```python
from build123d import *

# Parameters (mm, degrees)
SKETCH1_W           = 22
SKETCH1_H           = 14
BOSS_EXTRUDE1_DEPTH = 40
BOSS_EXTRUDE2_DEPTH = 5
SKETCH3_R           = 3.25
CUT_EXTRUDE1_DEPTH  = 41
SKETCH4_W           = 1.2
SKETCH4_H           = 40
CUT_EXTRUDE2_DEPTH  = 0.8


with BuildPart() as part:
    # Sketch1 → Boss-Extrude1 (new body)
    with BuildSketch(Plane(origin=(0, 0, 0), x_dir=(1, 0, 0), z_dir=(0, 1, 0))):
        with Locations((11, 7)):
            Rectangle(SKETCH1_W, SKETCH1_H)
    extrude(amount=BOSS_EXTRUDE1_DEPTH)

    # Sketch2 → Boss-Extrude2 (add)
    with BuildSketch(Plane(origin=(0, 40, 0), x_dir=(1, 0, 0), z_dir=(0, 1, 0))):
        Polygon((22, 0), (22, 2), (2, 2), (2, 12), (22, 12), (22, 14), (0, 14), (0, 0), align=None)
    extrude(amount=BOSS_EXTRUDE2_DEPTH)

    # Sketch3 → Cut-Extrude1 (cut, through all)
    with BuildSketch(Plane(origin=(0, 40, 0), x_dir=(1, 0, 0), z_dir=(0, 1, 0))):
        with Locations((16.582903769, 7)):
            Circle(SKETCH3_R)
        Polygon((11.582903769, 7), (9.562177826, 10.5), (5.520725942, 10.5), (3.5, 7), (5.520725942, 3.5), (9.562177826, 3.5), align=None)
    extrude(amount=-CUT_EXTRUDE1_DEPTH, mode=Mode.SUBTRACT)

    # Sketch4 → Cut-Extrude2 (cut)
    with BuildSketch(Plane(origin=(22, 0, 0), x_dir=(0, 0, -1), z_dir=(1, 0, 0))):
        with Locations((7, 20)):
            Rectangle(SKETCH4_W, SKETCH4_H)
    extrude(amount=-CUT_EXTRUDE2_DEPTH, mode=Mode.SUBTRACT)


solid = part.part
```
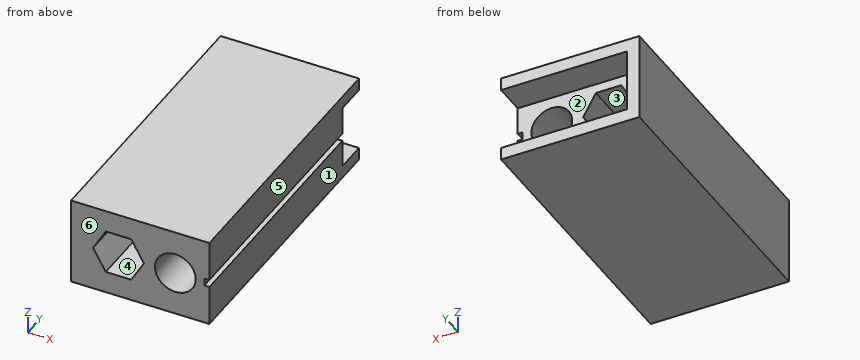
Could you check a few things on this model? Use its own coordinates, in mm. Face numbers are marked on the shaded views. A direction names the side the tool comes from. Give positions to 0.01 mm unless a question says otherwise; leave off trailing zeros. Loops run counter-clockwise (first coordinate to the right, second up) from the corner with the lowest first, then second, coordinate; pieces in that order, holes last. Notation, with made-up numbers: (61.25, -18.5) -> (85.25, -18.5) arc R15 ccw to (85.25, -4.5) -> close; hole circle Ø8 at (66, -6). An arc over 180 degrees is marked (long way). Put each result on its own line as item: value.
(1) I'm going to push flat-ended pins straight in: pin 1 Ø4 at (x, z) = (14.5, -5) entering from -Y; pin 2 Ø1.5 at (y, z) = (43.5, -4.5) entering from +X; pin 3 Ø0.6 at (y, z) = (24, -7) entering from +X; pin 4 Ø3 at (x, z) = (14.5, -5.5) entering from +Y. Where does each tip first touch, or does it pass through?
Computed:
pin 1: y = 0
pin 2: x = 2
pin 3: x = 21.2
pin 4: y = 40
(2) Imagine slicing it at B-B on x = 12.25. Write out the boundary of the cut face in (y, z).
Computed:
outline: (0, -14) -> (45, -14) -> (45, -12) -> (40, -12) -> (40, -2) -> (45, -2) -> (45, 0) -> (0, 0) -> close
(3) Imagine slicing it at A-A on y = 14.5. Write out the boundary of the cut face in (x, z).
Computed:
outline: (0, -14) -> (22, -14) -> (22, -7.6) -> (21.2, -7.6) -> (21.2, -6.4) -> (22, -6.4) -> (22, 0) -> (0, 0) -> close; hole (3.5, -7) -> (5.52, -10.5) -> (9.56, -10.5) -> (11.58, -7) -> (9.56, -3.5) -> (5.52, -3.5) -> close; hole circle Ø6.5 at (16.58, -7)
(4) For the marked faces 1, 2 and 3, which set-ups out of +Z, -Z, +X, -X, +Y, -Y let a thin tool reach every point of the face, with its end or its side?
Computed:
face 1: +Z, -Z, +X, +Y, -Y
face 2: +X, +Y
face 3: +Y, -Y
(5) Imagine slicing it at C-C on z = -5.25. Write out the boundary of the cut face in (x, y).
Computed:
outline: (0, 0) -> (4.51, 0) -> (4.51, 40) -> (2, 40) -> (2, 45) -> (0, 45) -> close; (10.57, 0) -> (13.84, 0) -> (13.84, 40) -> (10.57, 40) -> close; (19.32, 0) -> (22, 0) -> (22, 40) -> (19.32, 40) -> close
(6) Please list where these lines run through material, in increasing order: probe 1 along X at (y, z) = (19.5, -7); probe 2 along X at (y, z) = (34.5, -7.25); probe 3 along Z at (x, y) = (11.5, 41). Write a range as [from, to].
Computed:
probe 1: [0, 3.5], [11.58, 13.33], [19.83, 21.2]
probe 2: [0, 3.64], [11.44, 13.34], [19.82, 21.2]
probe 3: [-14, -12], [-2, 0]
(7) Thinking about a two-plate mould opening in X: for the marked faces 4, 5 and 6, which applies, pulls with the +X half, pulls with the -X half, needs draft (parallel to the pull), parting line crosses it, or undercut?
Computed:
face 4: undercut
face 5: pulls with the +X half
face 6: needs draft
(8) Imagine slicing it at D-D on x = 18. Write out the boundary of the cut face in (y, z), plus the area to 3 significant figures.
Computed:
outline: (0, -14) -> (45, -14) -> (45, -12) -> (40, -12) -> (40, -9.92) -> (0, -9.92) -> close; (0, -4.08) -> (40, -4.08) -> (40, -2) -> (45, -2) -> (45, 0) -> (0, 0) -> close
area: 346 mm^2
